```python
from build123d import *

# Parameters (mm, degrees)
SKETCH_1_W         = 266
SKETCH_1_H         = 196
SKETCH_1_R         = 2.25
EXTRUDE_1_DEPTH    = 3
SKETCH1_W          = 218
SKETCH1_H          = 38
CUT_EXTRUDE1_DEPTH = 4
FILLET1_R          = 3


with BuildPart() as part:
    # Эскиз1 → Бобышка-Вытянуть1 (new body)
    with BuildSketch(Plane(origin=(0, 0, 0), x_dir=(1, 0, 0), z_dir=(0, 1, 0))):
        with Locations((133, 98)):
            Rectangle(SKETCH_1_W, SKETCH_1_H)
        with Locations((13, 183)):
            Circle(SKETCH_1_R, mode=Mode.SUBTRACT)
        with Locations((253, 183)):
            Circle(SKETCH_1_R, mode=Mode.SUBTRACT)
        with Locations((253, 13)):
            Circle(SKETCH_1_R, mode=Mode.SUBTRACT)
        with Locations((13, 13)):
            Circle(SKETCH_1_R, mode=Mode.SUBTRACT)
        with Locations((133, 13)):
            Circle(SKETCH_1_R, mode=Mode.SUBTRACT)
        with Locations((133, 183)):
            Circle(SKETCH_1_R, mode=Mode.SUBTRACT)
    extrude(amount=EXTRUDE_1_DEPTH)

    # Sketch1 → Cut-Extrude1 (cut, through all)
    with BuildSketch(Plane.XZ):
        with Locations((133, -43)):
            Rectangle(SKETCH1_W, SKETCH1_H)
    extrude(amount=-CUT_EXTRUDE1_DEPTH, mode=Mode.SUBTRACT)

    # Fillet1
    fillet1_edges = [part.edges().sort_by_distance(p)[0] for p in [
        (24, 1.5, -62),
        (24, 1.5, -24),
        (242, 1.5, -24),
        (242, 1.5, -62),
    ]]
    fillet(fillet1_edges, radius=FILLET1_R)


solid = part.part
```
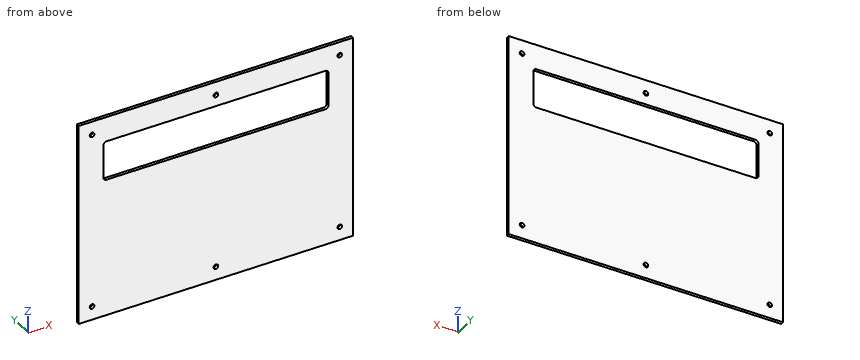
Check sheet for the modelled part. Datum: model origin and axes. Units: mm. Give positions to 0.01 mm unless a question says otherwise; leave off trailing zeros. Write each loop counter-clockwise with the first axis right and the second up, starting at its lowest first coordinate (ties: lowest second). Pieces come first, ordered by that corner, then holes. Notation, with made-up numbers: (52.25, 74) -> (83.25, 74) arc R10 cw to (83.25, 79) -> close; hole circle Ø5 at (5, 28). An arc over 180 degrees is marked (long way). Use CSV: the item, a comma, the result in double quotes. Start each with the question number.
Q1. Depth check by flat-ended pin: P1, Ø3.5, axis at x = 253, z = -183, coming from the +Y side. Enter the tip coordinate at first touch or a pass-through.
Q2. Scan lines: line 1 along Z through (x, y) = (253, 2.3); line 2 along X through (y, z) = (1.05, -183); line 3 along Z through (x, y) = (70.5, 1.6). Record each from-to range of solid material in increasing order.
Q3. Cross-section at B-B on y = 0.75. Enter the section's corners in (x, z).
Q4. Cross-section at A-A on x = 77.5. Enter the section's corners in (y, z).
Working result:
1,P1,"passes through"
2,line 1,"z = -196 to -185.25, -180.75 to -15.25, -10.75 to 0"
2,line 2,"x = 0 to 10.75, 15.25 to 130.75, 135.25 to 250.75, 255.25 to 266"
2,line 3,"z = -196 to -62, -24 to 0"
3,outline,"(0, -196) -> (266, -196) -> (266, 0) -> (0, 0) -> close; hole circle Ø4.5 at (13, -183); hole circle Ø4.5 at (13, -13); hole (24, -59) arc R3 ccw to (27, -62) -> (239, -62) arc R3 ccw to (242, -59) -> (242, -27) arc R3 ccw to (239, -24) -> (27, -24) arc R3 ccw to (24, -27) -> close; hole circle Ø4.5 at (133, -183); hole circle Ø4.5 at (133, -13); hole circle Ø4.5 at (253, -183); hole circle Ø4.5 at (253, -13)"
4,outline,"(0, -196) -> (3, -196) -> (3, -62) -> (0, -62) -> close; (0, -24) -> (3, -24) -> (3, 0) -> (0, 0) -> close"
